from build123d import *

# Parameters (mm, degrees)
SKETCH1_W           = 40
SKETCH1_H           = 24
BOSS_EXTRUDE1_DEPTH = 2
SKETCH2_W           = 40
SKETCH2_H           = 24
SKETCH2_W_2         = 36
SKETCH2_H_2         = 22
BOSS_EXTRUDE3_DEPTH = 8
SKETCH5_W           = 4
SKETCH5_H           = 3
CUT_EXTRUDE1_DEPTH  = 2
SKETCH6_W           = 24
SKETCH6_H           = 10
CUT_EXTRUDE2_DEPTH  = 2
SKETCH7_W           = 22
SKETCH7_H           = 8
CUT_EXTRUDE3_DEPTH  = 2
SKETCH8_W           = 1
SKETCH8_H           = 3
CUT_EXTRUDE4_DEPTH  = 2
SKETCH9_W           = 38
SKETCH9_H           = 24
CUT_EXTRUDE5_DEPTH  = 9
SKETCH10_W          = 38
SKETCH10_H          = 1
CUT_EXTRUDE6_DEPTH  = 0.25
SKETCH11_W          = 38
SKETCH11_H          = 1
CUT_EXTRUDE7_DEPTH  = 0.25


with BuildPart() as part:
    # Sketch1 → Boss-Extrude1 (new body)
    with BuildSketch(Plane(origin=(0, 0, 0), x_dir=(1, 0, 0), z_dir=(0, 1, 0))):
        with Locations((20, 12)):
            Rectangle(SKETCH1_W, SKETCH1_H)
    extrude(amount=BOSS_EXTRUDE1_DEPTH)

    # Sketch2 → Boss-Extrude3 (add)
    with BuildSketch(Plane(origin=(0, 2, 0), x_dir=(1, 0, 0), z_dir=(0, 1, 0))):
        with Locations((20, 12)):
            Rectangle(SKETCH2_W, SKETCH2_H)
        with Locations((21, 12)):
            Rectangle(SKETCH2_W_2, SKETCH2_H_2, mode=Mode.SUBTRACT)
    extrude(amount=BOSS_EXTRUDE3_DEPTH)

    # Sketch5 → Cut-Extrude1 (cut)
    with BuildSketch(Plane(origin=(0, 2, 0), x_dir=(1, 0, 0), z_dir=(0, 1, 0))):
        with Locations((6, 2.5)):
            Rectangle(SKETCH5_W, SKETCH5_H)
    extrude(amount=-CUT_EXTRUDE1_DEPTH, mode=Mode.SUBTRACT)

    # Sketch6 → Cut-Extrude2 (cut)
    with BuildSketch(Plane(origin=(40, 0, 0), x_dir=(0, 0, -1), z_dir=(1, 0, 0))):
        with Locations((12, 5)):
            Rectangle(SKETCH6_W, SKETCH6_H)
    extrude(amount=-CUT_EXTRUDE2_DEPTH, mode=Mode.SUBTRACT)

    # Sketch7 → Cut-Extrude3 (cut)
    with BuildSketch(Plane(origin=(3, 0, 0), x_dir=(0, 0, -1), z_dir=(1, 0, 0))):
        with Locations((12, 6)):
            Rectangle(SKETCH7_W, SKETCH7_H)
    extrude(amount=-CUT_EXTRUDE3_DEPTH, mode=Mode.SUBTRACT)

    # Sketch8 → Cut-Extrude4 (cut)
    with BuildSketch(Plane(origin=(0, 2, 0), x_dir=(1, 0, 0), z_dir=(0, 1, 0))):
        with Locations((3.5, 2.5)):
            Rectangle(SKETCH8_W, SKETCH8_H)
    extrude(amount=-CUT_EXTRUDE4_DEPTH, mode=Mode.SUBTRACT)

    # Sketch9 → Cut-Extrude5 (cut)
    with BuildSketch(Plane(origin=(0, 10, 0), x_dir=(1, 0, 0), z_dir=(0, 1, 0))):
        with Locations((19, 12)):
            Rectangle(SKETCH9_W, SKETCH9_H)
    extrude(amount=-CUT_EXTRUDE5_DEPTH, mode=Mode.SUBTRACT)

    # Sketch10 → Cut-Extrude6 (cut)
    with BuildSketch(Plane.XY):
        with Locations((19, 0.5)):
            Rectangle(SKETCH10_W, SKETCH10_H)
    extrude(amount=-CUT_EXTRUDE6_DEPTH, mode=Mode.SUBTRACT)

    # Sketch11 → Cut-Extrude7 (cut)
    with BuildSketch(Plane(origin=(0, 0, -24), x_dir=(-1, 0, 0), z_dir=(0, 0, -1))):
        with Locations((-19, 0.5)):
            Rectangle(SKETCH11_W, SKETCH11_H)
    extrude(amount=-CUT_EXTRUDE7_DEPTH, mode=Mode.SUBTRACT)


solid = part.part
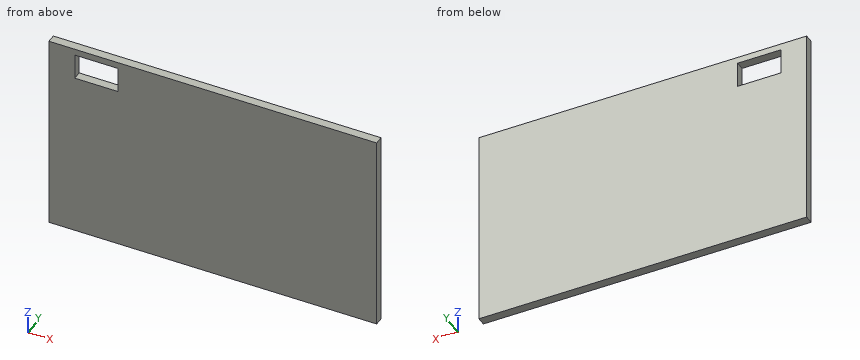
Input: part model. Units: mm. Frame: model coordinates. Round coordinates to 2 decimals unless told otherwise and drop trailing zeros. Loops run counter-clockwise (first coordinate to the right, second up) from the corner with the lowest first, then second, coordinate; pieces in that order, holes last. Notation, with made-up numbers: M 22.25,25 L 43.25,25 A26 ccw 43.25,44 Z; hole C 46,86 d6. An arc over 180 degrees is marked long. Answer as CSV lines item,"result". Start each with the question number.
(1) Line query: line 1 (Z direction, x = 7, y = 0.8); line 2 (X direction, y = 0.4, z = -3.5). Output: solid intervals per line, ascending. Write a range as [from, to].
(2) Section B-B, the plane x = 7. Output: boundary loops of the cut face in (y, z), plus the area to 3 significant figures.
(3) Section A-A, the plane y = 0.2. Output: boundary loops of the cut face in (x, z), plus the area to 3 significant figures.
Values found:
1,line 1,"z = [-23.75, -4], [-1, -0.25]"
1,line 2,"x = [0, 3], [8, 38]"
2,outline,"M 0,-23.75 L 1,-23.75 L 1,-4 L 0,-4 Z; M 0,-1 L 1,-1 L 1,-0.25 L 0,-0.25 Z"
2,area,"20.5 mm²"
3,outline,"M 0,-23.75 L 38,-23.75 L 38,-0.25 L 0,-0.25 Z; hole M 3,-4 L 8,-4 L 8,-1 L 3,-1 Z"
3,area,"878 mm²"
